Read the model definition and answer for the solid it produces. Units are mm, in the model's axes. Face numbers are marked on the shaded views. A direction names the side the tool comes from. Coordinates: 2 decimals unless noted, no trailing zeros. Order: outer loops, then holes, each group sorted by start corner. A loop starts at its lowest first (then second) coordinate and runs counter-clockwise, first axis right, second up.
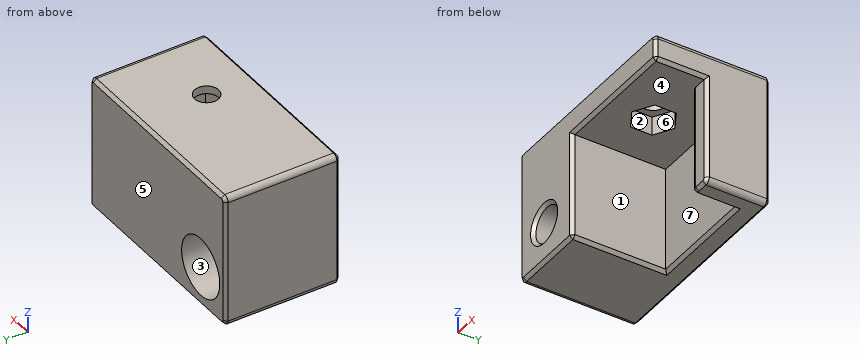
```python
from build123d import *

# Parameters (mm, degrees)
BOSS_EXTRUDE1_DEPTH                                 = 7.5
CBORE_FOR_M6_HEX_SOCKET_HEAD_CAP_SCREW1_D           = 6.6
CBORE_FOR_M6_HEX_SOCKET_HEAD_CAP_SCREW1_CBORE_D     = 11
CBORE_FOR_M6_HEX_SOCKET_HEAD_CAP_SCREW1_CBORE_DEPTH = 9
BOSS_EXTRUDE2_DEPTH                                 = 5
SKETCH6_W                                           = 39
SKETCH6_H                                           = 21.6
BOSS_EXTRUDE3_DEPTH                                 = 5
CUT_EXTRUDE1_DEPTH                                  = 3.5
M4_CLEARANCE_HOLE1_D                                = 4.5
FILLET1_R                                           = 1
CHAMFER1_SIZE                                       = 0.6


with BuildPart() as part:
    # Sketch1 → Boss-Extrude1 (new, symmetric)
    with BuildSketch(Plane.XY):
        Polygon((0, 0), (0, 21.6), (39, 21.6), (39, 9.6), (35, 9.6), (35, 17.6), (15, 17.6), (15, 0), align=None)
    extrude(amount=BOSS_EXTRUDE1_DEPTH, both=True)

    # CBORE for M6 Hex Socket Head Cap Screw1 (through all)
    with Locations(Plane(origin=(0, 21.6, 0), x_dir=(1, 0, 0), z_dir=(0, 1, 0))):
        with Locations((7, 0)):
            CounterBoreHole(CBORE_FOR_M6_HEX_SOCKET_HEAD_CAP_SCREW1_D / 2, CBORE_FOR_M6_HEX_SOCKET_HEAD_CAP_SCREW1_CBORE_D / 2, CBORE_FOR_M6_HEX_SOCKET_HEAD_CAP_SCREW1_CBORE_DEPTH)

    # Sketch5 → Boss-Extrude2 (add)
    with BuildSketch(Plane.XY.offset(7.5)):
        Polygon((0, 0), (15, 0), (15, 17.6), (35, 17.6), (35, 9.6), (39, 9.6), (39, 21.6), (0, 21.6), align=None)
    extrude(amount=BOSS_EXTRUDE2_DEPTH)

    # Sketch6 → Boss-Extrude3 (add)
    with BuildSketch(Plane.XY.offset(12.5)):
        with Locations((19.5, 10.8)):
            Rectangle(SKETCH6_W, SKETCH6_H)
    extrude(amount=BOSS_EXTRUDE3_DEPTH)

    # Sketch7 → Cut-Extrude1 (cut)
    with BuildSketch(Plane(origin=(0, 0, 12.5), x_dir=(-1, 0, 0), z_dir=(0, 0, -1))):
        Polygon((-25, 4.758548116), (-21.5, 6.779274058), (-21.5, 10.820725942), (-25, 12.841451884), (-28.5, 10.820725942), (-28.5, 6.779274058), align=None)
    extrude(amount=-CUT_EXTRUDE1_DEPTH, mode=Mode.SUBTRACT)

    # M4 Clearance Hole1 (through all)
    with Locations(Plane(origin=(0, 0, 16), x_dir=(-1, 0, 0), z_dir=(0, 0, -1))):
        with Locations((-25, 8.8)):
            Hole(M4_CLEARANCE_HOLE1_D / 2)

    # Fillet1
    fillet1_edges = [part.edges().sort_by_distance(p)[0] for p in [
        (35, 9.6, 2.5),
        (0, 10.8, 17.5),
        (39, 10.8, 17.5),
        (0, 10.8, -7.5),
        (39, 15.6, -7.5),
    ]]
    fillet(fillet1_edges, radius=FILLET1_R)

    # Chamfer1
    chamfer1_edges = [part.edges().sort_by_distance(p)[0] for p in [
        (0.292893219, 21.6, -7.207106781),
        (38.707106781, 21.6, 17.207106781),
        (35, 14.1, -7.5),
        (38.707106781, 21.6, -7.207106781),
        (8, 0, -7.5),
        (37, 9.6, -7.5),
        (35.292893219, 9.892893219, -7.5),
        (25, 17.6, -7.5),
        (38.707106781, 9.6, -7.207106781),
        (19.5, 0, 17.5),
        (0, 0, 5),
        (15, 8.8, -7.5),
        (0.292893219, 0, 17.207106781),
        (0.292893219, 0, -7.207106781),
        (38.707106781, 0, 17.207106781),
        (39, 9.6, 3),
        (15, 0, 2.5),
        (10.3, 0, 0),
        (27, 0, 12.5),
        (39, 4.8, 12.5),
        (39, 21.6, 5),
        (39, 0, 14.5),
        (19.5, 21.6, -7.5),
        (0, 21.6, 5),
        (19.5, 21.6, 17.5),
        (0.292893219, 21.6, 17.207106781),
    ]]
    chamfer(chamfer1_edges, length=CHAMFER1_SIZE)


solid = part.part
```
1) A cutting plane is placed at C-C, the plane x = 7. Determine the outline of the cut face in (y, z).
A:
outline: (0, -6.9) - (0.6, -7.5) - (21, -7.5) - (21.6, -6.9) - (21.6, -5.5) - (12.6, -5.5) - (12.6, -3.3) - (0.6, -3.3) - (0, -3.9) - close; (0, 3.9) - (0.6, 3.3) - (12.6, 3.3) - (12.6, 5.5) - (21.6, 5.5) - (21.6, 16.9) - (21, 17.5) - (0.6, 17.5) - (0, 16.9) - close
2) A cutting plane is placed at A-A, the plane y = 8.8. Determine the outline of the cut face in (x, z), and give its area (3 significant figures).
A:
outline: (0, -6.5) arc R1 ccw to (1, -7.5) - (14.4, -7.5) - (15, -6.9) - (15, 12.5) - (21.5, 12.5) - (21.5, 16) - (22.75, 16) - (22.75, 17.5) - (1, 17.5) arc R1 ccw to (0, 16.5) - close; (27.25, 16) - (28.5, 16) - (28.5, 12.5) - (38.4, 12.5) - (39, 13.1) - (39, 16.5) arc R1 ccw to (38, 17.5) - (27.25, 17.5) - close; hole circle Ø6.6 at (7, 0)
area: 429 mm2
3) Straight lines are drawn through the part: line 1 (X direction, y = 11.5, z = 0.25); line 2 (X direction, y = 3.25, z = 0); line 3 (Z direction, x = 7, y = 3.75). For each, find the intervals that lie inside material, in ascending order.
A:
line 1: x = 0 to 3.71, 10.29 to 15, 35 to 39
line 2: x = 0 to 3.7, 10.3 to 15
line 3: z = -7.5 to -3.3, 3.3 to 17.5
4) Which of the six approach directions +Z, -Z, +X, -X, +Y, -Y give full straight-line access (tool end or side, diameter ignored) to the marked faces 1, 2 and 3?
A:
face 1: -Z, -Y
face 2: -Z
face 3: +Y
5) A cutting plane is placed at D-D, the plane z = 7.5. Determine the outline of the cut face in (x, y).
A:
outline: (0, 0.6) - (0.6, 0) - (14.4, 0) - (15, 0.6) - (15, 17.6) - (35, 17.6) - (35, 10.6) arc R1 ccw to (36, 9.6) - (38.4, 9.6) - (39, 10.2) - (39, 21) - (38.4, 21.6) - (0.6, 21.6) - (0, 21) - close
6) A cutting plane is placed at B-B, the plane z = 0. Determine the outline of the cut face in (x, y).
A:
outline: (0, 0.6) - (0.6, 0) - (3.1, 0) - (3.7, 0.6) - (3.7, 12.6) - (1.5, 12.6) - (1.5, 21.6) - (0.6, 21.6) - (0, 21) - close; (10.3, 0.6) - (10.9, 0) - (14.4, 0) - (15, 0.6) - (15, 17.6) - (35, 17.6) - (35, 10.6) arc R1 ccw to (36, 9.6) - (38.4, 9.6) - (39, 10.2) - (39, 21) - (38.4, 21.6) - (12.5, 21.6) - (12.5, 12.6) - (10.3, 12.6) - close
7) Determine the mould class of the marked faces 4, 5, 6 and 7 for opening direction Y: pulls with the +Y half, pulls with the -Y half, needs draft (parallel to the pull), parting line crosses it, or undercut.
A:
face 4: needs draft
face 5: pulls with the +Y half
face 6: undercut
face 7: pulls with the -Y half
8) Flat-ended cylindrical pins translate along their axes: pin 1 Ø5 at (x, y) = (32, 7) entering from -Z; pin 2 Ø1.9 at (x, z) = (37.5, 0.5) entering from -Y; pin 3 Ø2.5 at (x, y) = (25, 8.8) entering from +Z; pin 4 Ø5.5 at (x, z) = (5, 0.5) entering from +Y. Find the tip coordinate at first contact, or state that the pin passes through.
A:
pin 1: stops at z = 12.5
pin 2: stops at y = 9.6
pin 3: passes through
pin 4: stops at y = 12.6
